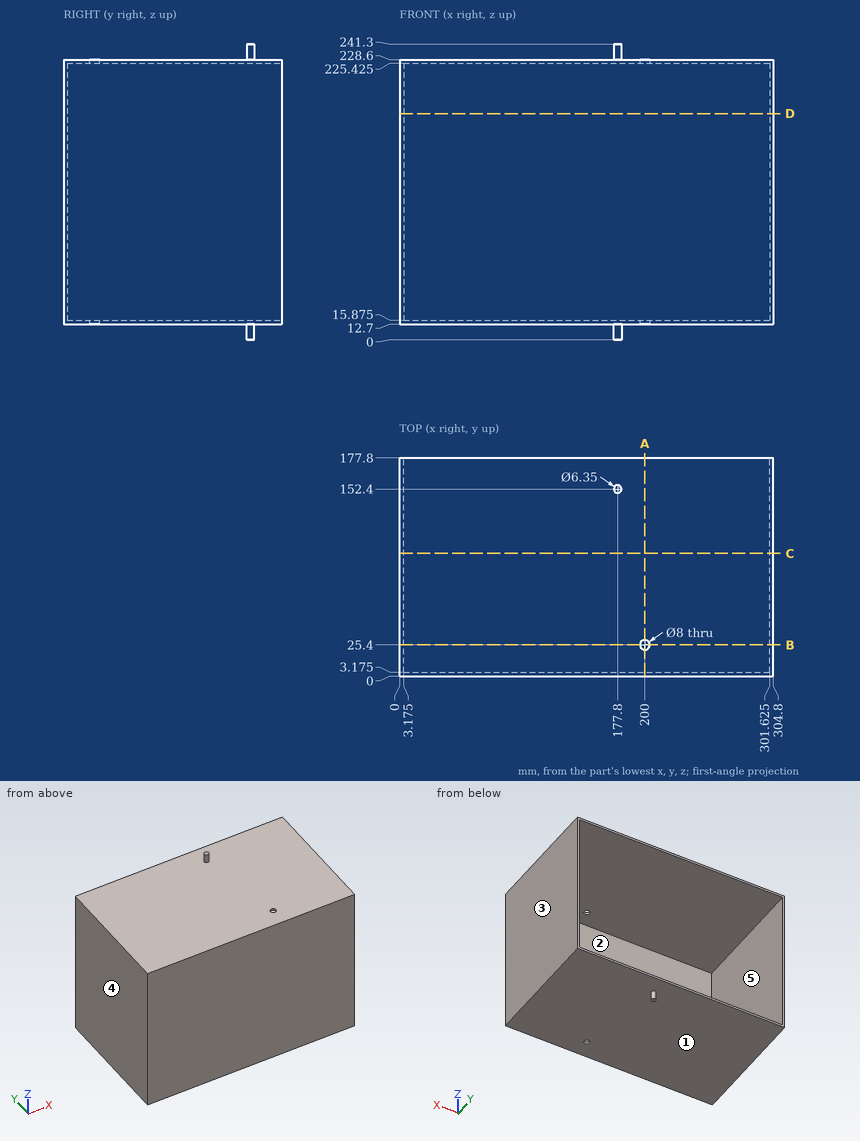
Answer from the drawing. Dimensions are ordinates in mm from the lowest x, y and z of the part. A direction names the side the tool comes from. Coordinates: 2 decimals unless noted, no trailing zeros. Loops run counter-clockwise (first coordinate to the right, second up) from the corner with the lowest first, then second, coordinate; pieces in that order, holes last. Notation, with made-up numbers: (78.5, 51.25) -> (104.5, 51.25) arc R31 ccw to (104.5, 89.25) -> close; hole circle Ø9 at (-18.5, 67.5). An arc over 180 degrees is marked (long way). Answer as CSV lines item,"result".
Q1. The part is cut by section A-A on x = 200. Write down the section's boundary in (y, z) (3 decimals).
Findings:
outline,"(0, 12.7) -> (21.4, 12.7) -> (21.4, 15.875) -> (3.175, 15.875) -> (3.175, 225.425) -> (21.4, 225.425) -> (21.4, 228.6) -> (0, 228.6) -> close; (29.4, 12.7) -> (177.8, 12.7) -> (177.8, 15.875) -> (29.4, 15.875) -> close; (29.4, 225.425) -> (177.8, 225.425) -> (177.8, 228.6) -> (29.4, 228.6) -> close"
Q2. Each of these flat-tipped pins is pushed along its axis until it touches: pin 1 (4 mm diameter, centred on x = 114, y = 38.5, fed in from -Z); pin 2 (6 mm diameter, centred on x = 159.5, y = 115, fed in from +Z); pin 3 (6 mm diameter, centred on x = 257.5, z = 192, fed in from +Y) (3 decimals); pin 4 (7 mm diameter, centred on x = 200, y = 25.4, fed in from +Z). Where does it stop, or does it pass through?
Findings:
pin 1,"stops at z = 12.7"
pin 2,"stops at z = 228.6"
pin 3,"stops at y = 3.175"
pin 4,"passes through"
Q3. Find the intervals of material crossed by probe 1 along Z at (x, y) = (133, 148) (3 decimals); probe 2 along X at (y, z) = (124.5, 60) (3 decimals); probe 3 along Y at (x, z) = (200, 14), in increasing order.
Findings:
probe 1,"z = 12.7 to 15.875, 225.425 to 228.6"
probe 2,"x = 0 to 3.175, 301.625 to 304.8"
probe 3,"y = 0 to 21.4, 29.4 to 177.8"
Q4. The part is cut by section B-B on y = 25.4. Write down the section's boundary in (x, z) (3 decimals).
Findings:
outline,"(0, 12.7) -> (196, 12.7) -> (196, 15.875) -> (3.175, 15.875) -> (3.175, 225.425) -> (196, 225.425) -> (196, 228.6) -> (0, 228.6) -> close; (204, 12.7) -> (304.8, 12.7) -> (304.8, 228.6) -> (204, 228.6) -> (204, 225.425) -> (301.625, 225.425) -> (301.625, 15.875) -> (204, 15.875) -> close"
Q5. A tool of negligible diameter and unlimited length cuts with its end or side. For the marked faces 4 and 5, from which of +Z, -Z, +X, -X, +Y, -Y can it reach the whole face along a straight path? Write none if from no direction.
Findings:
face 4,"+Z, -Z, -X, +Y, -Y"
face 5,"+Y"
Q6. The part is cut by section D-D on z = 184.5. Write down the section's boundary in (x, y) (3 decimals), and give its area (3 significant figures).
Findings:
outline,"(0, 0) -> (304.8, 0) -> (304.8, 177.8) -> (301.625, 177.8) -> (301.625, 3.175) -> (3.175, 3.175) -> (3.175, 177.8) -> (0, 177.8) -> close"
area,"2,080 mm²"
Q7. The part is cut by section C-C on y = 100. Write down the section's boundary in (x, z) (3 decimals), and give its area (3 significant figures).
Findings:
outline,"(0, 12.7) -> (304.8, 12.7) -> (304.8, 228.6) -> (0, 228.6) -> close; hole (3.175, 15.875) -> (301.625, 15.875) -> (301.625, 225.425) -> (3.175, 225.425) -> close"
area,"3,270 mm²"
Q8. For a pull along X with two mould halves and no side action, classify the marked faces 1, 2 and 3 as +X half, -X half, draft (parallel to the pull), parting line (faces both ways), or undercut.
Findings:
face 1,"draft"
face 2,"undercut"
face 3,"+X half"
